The drawing under review shows one solid part. Ordinate dimensions are in mm from its lowest x, y, z. A direction names the side the tool comes from. Coordinates: 2 decimals unless noted, no trailing zeros. Write each loop counter-clockwise with the first axis right and the second up, starting at its lowest first coordinate (ties: lowest second). Pieces come first, ordered by that corner, then holes.
Q1. Clearance check with flat-ended pins moving along their axes: pin 1 Ø2.5 at (x, z) = (86, 3.5) entering from -Y (1 decimal); pin 2 Ø8 at (y, z) = (11.5, 25.5) entering from +X; pin 3 Ø10 at (y, z) = (16, 11.5) entering from -X; pin 4 Ø2 at (x, y) = (97, 56.5) entering from +Z. State where each tip first meets the part, or that it passes through.
Q2. Add section D-D, the plane x = 116. Give the boundary of the cut face in (y, z).
Q3. To check wall thickness, follow probe 1 along X at (y, z) = (44, 4) (1 decimal); probe 2 along X at (y, z) = (87.25, 44.45); probe 3 along Y at (x, z) = (55.5, 19). State the ranges of each line that lie inside material, in increasing order.
Q4. The part is to be moulded in two halves that separate along Y. For the marked faces 3, 4, 5 and 6, say which applies: +Y half, -Y half, draft (parallel to the pull), parting line (faces both ways), or undercut.
Q5. Add section C-C, the plane x = 31.5. Give the boundary of the cut face in (y, z) (1 decimal), plus the area to 3 significant figures.
Q6. Machinability: for the marked faces 1 and 2, which of the approach directions +Z, -Z, +X, -X, +Y, -Y give a long, thin tool a straight path to every point of the face, cutting with its end or side? Answer none if there is none.
Q7. Add section B-B, the plane y = 43. Give the boundary of the cut face in (x, z).
Q8. Add section A-A, the plane z = 27. Give the boundary of the cut face in (x, y).
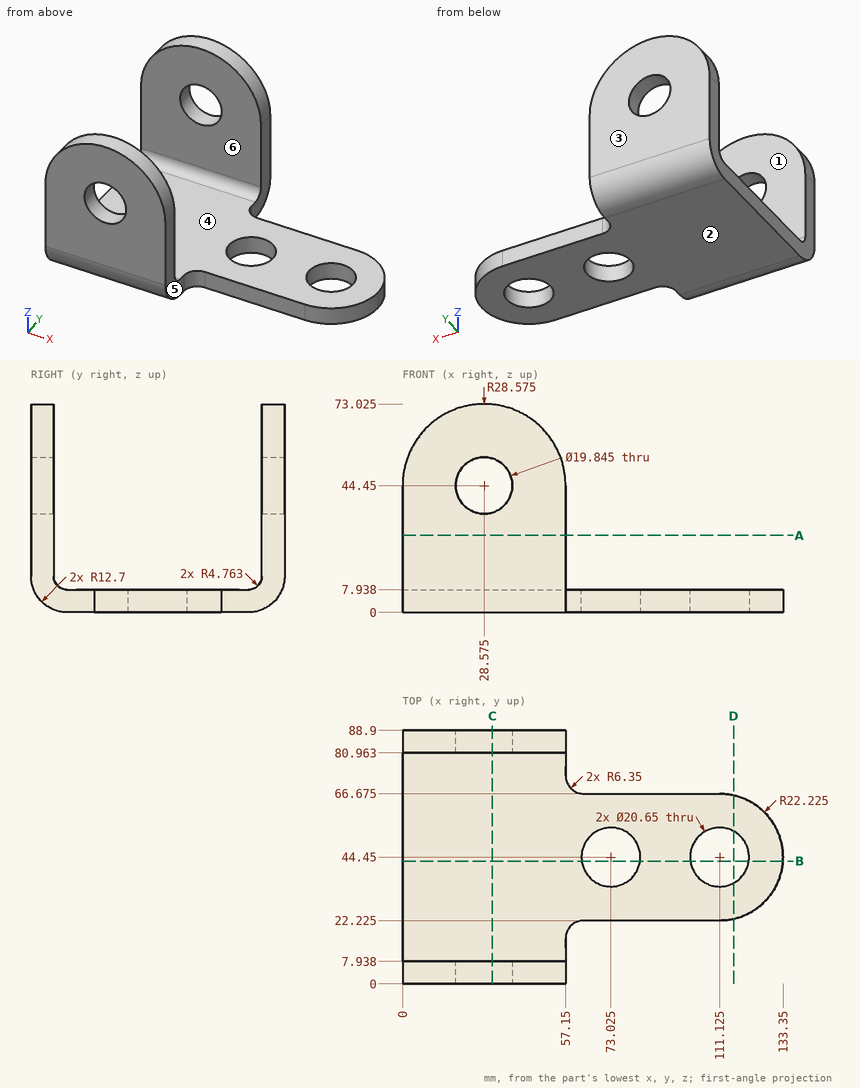
Here are the results:
1. pin 1: stops at y = 22.2
1. pin 2: stops at x = 57.15
1. pin 3: stops at x = 0
1. pin 4: stops at z = 7.94
2. outline: (22.77, 0) - (35.35, 0) - (35.35, 7.94) - (22.77, 7.94) - close; (53.55, 0) - (66.13, 0) - (66.13, 7.94) - (53.55, 7.94) - close
3. probe 1: x = 0 to 62.7, 83.3 to 100.8, 121.4 to 133.3
3. probe 2: x = 0 to 18.65, 38.5 to 57.15
3. probe 3: y = 0 to 7.94, 80.96 to 88.9
4. face 3: +Y half
4. face 4: undercut
4. face 5: draft
4. face 6: undercut
5. outline: (0, 12.7) arc R12.7 ccw to (12.7, 0) - (76.2, 0) arc R12.7 ccw to (88.9, 12.7) - (88.9, 35) - (81, 35) - (81, 12.7) arc R4.8 cw to (76.2, 7.9) - (12.7, 7.9) arc R4.8 cw to (7.9, 12.7) - (7.9, 35) - (0, 35) - close; (0, 53.9) - (7.9, 53.9) - (7.9, 72.9) - (0, 72.9) - close; (81, 53.9) - (88.9, 53.9) - (88.9, 72.9) - (81, 72.9) - close
5. area: 1,380 mm2
6. face 1: +Z, +X, -X
6. face 2: -Z, +X, -X, +Y, -Y
7. outline: (0, 0) - (62.8, 0) - (62.8, 7.94) - (0, 7.94) - close; (83.25, 0) - (100.9, 0) - (100.9, 7.94) - (83.25, 7.94) - close; (121.35, 0) - (133.3, 0) - (133.3, 7.94) - (121.35, 7.94) - close
8. outline: (0, 0) - (57.15, 0) - (57.15, 7.94) - (0, 7.94) - close; (0, 80.96) - (57.15, 80.96) - (57.15, 88.9) - (0, 88.9) - close
